Can you work these out from the model? Positions are in its coordinate system, mm. A direction names the side the tool comes from. Round coordinates to 2 decimals unless told otherwise and drop trailing zeros. Order: outer loops, then holes, each group sorted by start corner. A loop starts at its lowest first (then second) coordinate and runs counter-clockwise, first axis right, second up. Notation, with made-up numbers: (-28.5, -32.75) -> (27.5, -32.75) arc R30 cw to (27.5, -6.75) -> close; hole circle Ø4 at (-28.75, 80.5). An arc over 180 degrees is marked (long way). One line per item, written item: value.
```python
from build123d import *

# Parameters (mm, degrees)
SKETCH1_R           = 70
BOSS_EXTRUDE1_DEPTH = 30
BOSS_EXTRUDE2_DEPTH = 30
BOSS_EXTRUDE3_DEPTH = 30
CIRPATTERN1_COUNT   = 20


with BuildPart() as part:
    # Sketch1 → Boss-Extrude1 (new body)
    with BuildSketch(Plane(origin=(0, 0, 0), x_dir=(1, 0, 0), z_dir=(0, 1, 0))):
        Circle(SKETCH1_R)
    extrude(amount=BOSS_EXTRUDE1_DEPTH)

    # Sketch2 → Boss-Extrude2 (add)
    with BuildSketch(Plane(origin=(0, 0, 0), x_dir=(1, 0, 0), z_dir=(0, 1, 0))):
        Polygon((-5, 0), (5, 0), (5, 10), (0, 18.9908378), (-5, 10), align=None)
    extrude(amount=-BOSS_EXTRUDE2_DEPTH)

    # Sketch3 → Boss-Extrude3 (add)
    with BuildSketch(Plane(origin=(0, 30, 0), x_dir=(1, 0, 0), z_dir=(0, 1, 0))):
        with BuildLine():
            Line((0, 75), (0, 70))
            ThreePointArc((0, 70), (2.021982695, 69.970790949), (4.042277957, 69.883188171))
            Line((4.042277957, 69.883188171), (0, 75))
        make_face()
    boss_extrude3 = extrude(amount=-BOSS_EXTRUDE3_DEPTH)

    # CirPattern1: Boss-Extrude3 ×20 about axis
    cirpattern1_axis = Axis((0.000873645, 0, -0.046633798), (0, 1, 0))
    for i in range(1, CIRPATTERN1_COUNT):
        add(boss_extrude3.rotate(cirpattern1_axis, i * 360 / CIRPATTERN1_COUNT))


solid = part.part
```
Q1. Will these pins go through, and if not, where does the flat tip stop? pin 1 Ø10 at (x, y) = (-26, -8) entering from +Z; pin 2 Ø5 at (y, z) = (-20, -7.5) entering from +X; pin 3 Ø2.5 at (y, z) = (18.5, 71.5) entering from +X; pin 4 Ø10 at (x, y) = (7, -6.5) entering from +Z.
Answers below:
pin 1: through
pin 2: x = 5
pin 3: x = 23.16
pin 4: z = 0
Q2. On a 3-axis mill with a long thin cutter (end or side, diameter ignored), from which of +Z, -Z, +X, -X, +Y, -Y can I reach the whole of each face in a straight line? I mean faces 5 (the face through (-68.765, 14.79, -13.092)), 6 (the face through (-2.465, -14.79, -14.558)), 7 (the face through (-22.4, 15.2, 68.9)), 8 (the face through (68.782, 14.79, 13.001)). Say none if no direction works.
Answers below:
face 5: -X, +Y, -Y
face 6: -Z, -X, -Y
face 7: +Z, +Y, -Y
face 8: +X, +Y, -Y
Q3. I want a section at B-B on z = -14. List the corners of the cut face in (x, y) for me.
Answers below:
outline: (-68.59, 0) -> (-2.78, 0) -> (-2.78, -30) -> (2.78, -30) -> (2.78, 0) -> (68.59, 0) -> (68.59, 30) -> (-68.59, 30) -> close
Q4. I want a section at C-C on x = -12.5. List the corners of the cut face in (y, z) for me.
Answers below:
outline: (0, -68.87) -> (30, -68.87) -> (30, 68.87) -> (0, 68.87) -> close
Q5. Please list where these lines run through material, in increasing order: line 1 along Y through (x, z) = (17.5, 36); line 2 along X through (y, z) = (-7, -7); line 3 along Z through (x, y) = (-37.5, 20.5).
Answers below:
line 1: 0 to 30
line 2: -5 to 5
line 3: -59.11 to 59.11
Q6. I want a section at A-A on y = -17. List the corners of the cut face in (x, z) for me.
Answers below:
outline: (-5, -10) -> (0, -18.99) -> (5, -10) -> (5, 0) -> (-5, 0) -> close
Q7. We'd pull the mould along Z, two halves only. Please class faces 1 (the face through (-33.662, 14.79, 61.375)), 2 (the face through (44.19, 15.21, -57.39)), 3 (the face through (58.7, 15.2, 42.6)), 4 (the face through (42.633, 15.21, 58.631)): released by +Z, released by -Z, zero draft, split by the parting line, or undercut.
Answers below:
face 1: released by +Z
face 2: released by -Z
face 3: undercut
face 4: undercut
Q8. I want a section at D-D on z = -35. List the corners of the cut face in (x, y) for me.
Answers below:
outline: (-60.62, 0) -> (60.62, 0) -> (60.62, 30) -> (-60.62, 30) -> close
